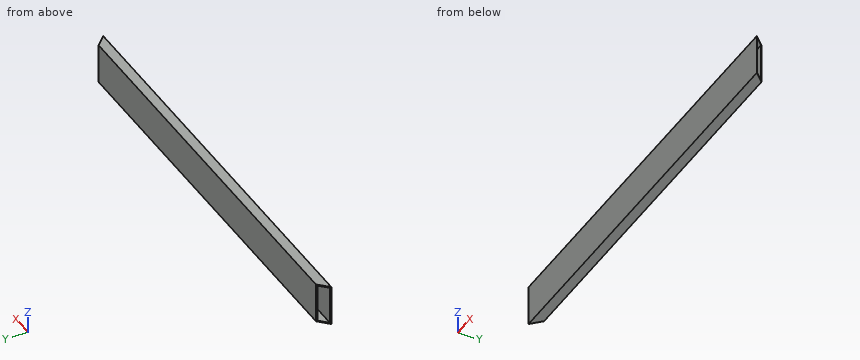
```python
from build123d import *

# Parameters (mm, degrees)
F0_W        = 50.8
F0_H        = 203.2
F0_W_2      = 41.275
F0_H_2      = 193.675
F1_DEPTH    = 2133.6
F2_T1_DEPTH = 464.4829915773
F3_T1_DEPTH = 464.4829915773


# Not quite as in the source:
# - a fillet or chamfer that OpenCascade refuses, or shapes differently, is made with other operations: its cross-section is extruded or revolved along the edge and cut away or added


with BuildPart() as f1:
    # F0 (on Right) → F1 (new body)
    with BuildSketch(Plane.YZ):
        with Locations((25.4, 101.6)):
            Rectangle(F0_W, F0_H)
        with Locations((25.4, 101.6)):
            Rectangle(F0_W_2, F0_H_2, mode=Mode.SUBTRACT)
    extrude(amount=-F1_DEPTH)

    # F2: chamfer of 50.8 on 1 edges, made by hand

    # F2_s2 → F2_t1 (cut)
    with BuildSketch(Plane.XY.offset(-130.6414957887)):
        Polygon((-50.8, 50.8), (0, 0), (0, 50.8), align=None)
    extrude(amount=F2_T1_DEPTH, mode=Mode.SUBTRACT)

    # F3: chamfer of 50.8 on 1 edges, made by hand

    # F3_s2 → F3_t1 (cut)
    with BuildSketch(Plane.XY.offset(-130.6414957887)):
        Polygon((-2133.6, 0), (-2082.8, 50.8), (-2133.6, 50.8), align=None)
    extrude(amount=F3_T1_DEPTH, mode=Mode.SUBTRACT)


solid = f1.part
```
Design review of the part built by this model. Coordinates are the model's own, in mm. Give positions to 0.01 mm unless a question says otherwise; leave off trailing zeros. Order: outer loops, then holes, each group sorted by start corner. A loop starts at its lowest first (then second) coordinate and runs counter-clockwise, first axis right, second up. Notation, with made-up numbers: (-1.75, -18.5) - (49.25, -18.5) arc R10 cw to (49.25, -9.5) - close; hole circle Ø10 at (-38.5, 75). An arc over 180 degrees is marked (long way). Use a Markdown table: item, result. Add a question column.
(1) Add section A-A on y = 38. Give the boundary of the cut face in (x, z).
(2) Add section B-B on z = 92. Give the boundary of the cut face in (x, y).
(3) Wall thickness on probe 1 along Y at (x, z) = (-1963, 176); probe 2 along Z at (x, y) = (-756, 36); probe 3 along X at (y, z) = (3.5, 39): over which ranges is each line inside the solid? List them lowest first. Write a range as [from, to].
(4) Add section C-C on x = -275. Give the boundary of the cut face in (y, z), then the cut area to 3 significant figures.
Report:
| question | item | result |
|---|---|---|
| 1 | outline | (-2095.6, 0) - (-38, 0) - (-38, 4.76) - (-2095.6, 4.76) - close; (-2095.6, 198.44) - (-38, 198.44) - (-38, 203.2) - (-2095.6, 203.2) - close |
| 2 | outline | (-2133.6, 0) - (0, 0) - (-4.76, 4.76) - (-2128.84, 4.76) - close; (-2087.56, 46.04) - (-46.04, 46.04) - (-50.8, 50.8) - (-2082.8, 50.8) - close |
| 3 | probe 1 | y = [0, 4.76], [46.04, 50.8] |
| 3 | probe 2 | z = [0, 4.76], [198.44, 203.2] |
| 3 | probe 3 | x = [-2130.1, -3.5] |
| 4 | outline | (0, 0) - (50.8, 0) - (50.8, 203.2) - (0, 203.2) - close; hole (4.76, 4.76) - (46.04, 4.76) - (46.04, 198.44) - (4.76, 198.44) - close |
| 4 | area | 2,330 mm² |
